Source: CAD feature listing. Evaluate the final solid. Frame: model axes, mm. A direction names the side the tool comes from. Give positions to 0.01 mm unless a question says otherwise; leave off trailing zeros. Loops run counter-clockwise (first coordinate to the right, second up) from the corner with the lowest first, then second, coordinate; pieces in that order, holes last. Notation, with made-up numbers: (-20, 24) -> (11, 24) arc R16 ccw to (11, 54) -> close; hole circle Ø6 at (76, 34). An arc over 180 degrees is marked (long way). Return JSON: item names as keys, results as strings. Group by question number.
(1) Cut plane A-A on y = 0.5. Return loops of the section in (x, z).
(2) Pin query (flat end, axial travel): pin 1 (3 mm diameter, centred on x = -4.5, y = 1, fed in from +Z); pin 2 (2 mm diameter, centred on y = -0.5, z = 1, fed in from -X); pin 3 (2 mm diameter, centred on x = -3.5, z = 2, fed in from +Y); pin 4 (1.1 mm diameter, centred on y = 0.5, z = 4.5, fed in from -X). Return the tip coordinate at first contact, or that it passes through.
(3) Draft query along X for faces 1 (the face through (-1.11, 0, 1)), 2 (the face through (-4.6, -1.684, 1.232)), 3 (the face through (-1.242, -3.219, 1.232)). Return one class per face: released by +X, released by -X, zero draft, split by the parting line, or undercut.
(4) Access query for faces 4 (the face through (-4.3, -1.4, 1.2)), 5 (the face through (0.9, 0.5, 7)), 6 (the face through (0.71, 0, 3)). Directions: +Z, -Z, +X, -X, +Y, -Y. A direction counts if a zero-diameter tool reaches every point of the face in a straight line with its end or side. Return the directions, or none.
(5) Ray query, line 1 (X direction, y = -0.75, z = 2); line 2 (X direction, y = -0.25, z = 3.25); line 3 (X direction, y = -1.25, z = 0.5). Return the intervals inside material, ascending. Write a range as from..to.
(6) Cut plane C-C on x = 0. Return loops of the section in (y, z) (3 decimals).
(7) Cut plane B-B on z = 0.5. Return loops of the section in (x, y) (3 decimals).
(8) Cut plane D-D on y = -2.5. Return loops of the section in (x, z), then the cut area to 3 significant figures.
```python
from build123d import *

# Parameters (mm, degrees)
BASE_FLANGE2_DEPTH  = 2.5
SKETCH10_W          = 0.4
SKETCH10_H          = 3.67
BOSS_EXTRUDE1_DEPTH = 4.5
SKETCH11_W          = 3.4
SKETCH11_H          = 1
CUT_EXTRUDE1_DEPTH  = 12.139958989
FILLET1_RADIUS      = 1.335
FILLET1_LENGTH      = 0.4


# Sheet-metal steps are written as plain solids
with BuildPart() as part:
    # Sketch1 → Base-Flange2 (new body)
    with BuildSketch(Plane.XY):
        with BuildLine():
            Line((-6.888528694, -0.229568793), (-2.246268811, -3.179047252))
            ThreePointArc((-2.246268811, -3.179047252), (-1.228475759, -3.211432773), (-0.71, -2.335))
            Line((-0.71, -2.335), (-0.71, -1.835))
            Line((-0.71, -1.835), (-0.71, 1.835))
            ThreePointArc((-0.71, 1.835), (0, 2.545), (0.71, 1.835))
            Line((0.71, 1.835), (0.71, -1.835))
            Line((0.71, -1.835), (1.11, -1.835))
            Line((1.11, -1.835), (1.11, 1.835))
            ThreePointArc((1.11, 1.835), (0, 2.945), (-1.11, 1.835))
            Line((-1.11, 1.835), (-1.11, -1.835))
            Line((-1.11, -1.835), (-1.11, -2.335))
            ThreePointArc((-1.11, -2.335), (-1.421085455, -2.860859664), (-2.031761286, -2.841428351))
            Line((-2.031761286, -2.841428351), (-6.67402117, 0.108050107))
            Line((-6.67402117, 0.108050107), (-6.888528694, -0.229568793))
        make_face()
    extrude(amount=BASE_FLANGE2_DEPTH)

    # Sketch10 → Boss-Extrude1 (add)
    with BuildSketch(Plane.XY.offset(2.5)):
        with Locations((0.91, 0)):
            Rectangle(SKETCH10_W, SKETCH10_H)
    extrude(amount=BOSS_EXTRUDE1_DEPTH)

    # Sketch11 → Cut-Extrude1 (cut, through all)
    with BuildSketch(Plane(origin=(1.11, 0, 0), x_dir=(0, 0, -1), z_dir=(1, 0, 0))):
        with Locations((-5.3, -1.335)):
            Rectangle(SKETCH11_W, SKETCH11_H)
    extrude(amount=-CUT_EXTRUDE1_DEPTH, mode=Mode.SUBTRACT)

    # Fillet1: full round fillet: the end face becomes a half cylinder, R = half its width
    fillet1_face = Plane((0.91, 0.5, 7), x_dir=(-1, 0, 0), z_dir=(0, 0, 1))  # on the end face: x along it, z out of the body
    fillet1_slab = fillet1_face.offset(-FILLET1_RADIUS / 2) * Box(FILLET1_LENGTH, 2 * FILLET1_RADIUS, FILLET1_RADIUS, mode=Mode.PRIVATE)  # the body's end, R deep
    fillet1_round = Plane((0.91, 0.5, 5.665), x_dir=(0, 0, 1), z_dir=(-1, 0, 0)) * Cylinder(FILLET1_RADIUS, FILLET1_LENGTH, mode=Mode.PRIVATE)  # its axis R under the face
    add(fillet1_slab - fillet1_round, mode=Mode.SUBTRACT)


solid = part.part
```
Answers:
{
 "1": {"outline": "(-1.11, 0) -> (-0.71, 0) -> (-0.71, 2.5) -> (-1.11, 2.5) -> close; (0.71, 0) -> (1.11, 0) -> (1.11, 7) -> (0.71, 7) -> close"},
 "2": {"pin 1": "through", "pin 2": "x = -6.89", "pin 3": "y = -1.27", "pin 4": "x = 0.71"},
 "3": {"face 1": "undercut", "face 2": "released by -X", "face 3": "split by the parting line"},
 "4": {"face 4": "+Z, -Z, +Y", "face 5": "+Z, +X, -X", "face 6": "+Z, -Z, -Y"},
 "5": {"line 1": "-6.07..-5.32, -1.11..-0.71, 0.71..1.11", "line 2": "0.71..1.11", "line 3": "-5.28..-4.54, -1.11..-0.71, 0.71..1.11"},
 "6": {"outline": "(2.545, 0) -> (2.945, 0) -> (2.945, 2.5) -> (2.545, 2.5) -> close"},
 "7": {"outline": "(-6.889, -0.23) -> (-2.246, -3.179) arc R1 ccw to (-0.71, -2.335) -> (-0.71, 1.835) arc R0.71 cw to (0.71, 1.835) -> (0.71, -1.835) -> (1.11, -1.835) -> (1.11, 1.835) arc R1.11 ccw to (-1.11, 1.835) -> (-1.11, -2.335) arc R0.6 cw to (-2.032, -2.841) -> (-6.674, 0.108) -> close"},
 "8": {"outline": "(-3.32, 0) -> (-2.57, 0) -> (-2.57, 2.5) -> (-3.32, 2.5) -> close; (-1.13, 0) -> (-0.72, 0) -> (-0.72, 2.5) -> (-1.13, 2.5) -> close", "area": "2.89 mm²"}
}
